from build123d import *

# Parameters (mm, degrees)
SKETCH1_R           = 37.5
SKETCH1_R_2         = 1.5
BOSS_EXTRUDE1_DEPTH = 10
FILLET1_R           = 5


with BuildPart() as part:
    # Sketch1 → Boss-Extrude1 (new body)
    with BuildSketch(Plane(origin=(0, 0, 0), x_dir=(1, 0, 0), z_dir=(0, 1, 0))):
        with Locations(Location((0, 0, 0), (0, 0, 270))):
            Circle(SKETCH1_R)
        with Locations(Location((-24.748737342, -24.748737342, 0), (0, 0, 270))):
            Circle(SKETCH1_R_2, mode=Mode.SUBTRACT)
        with Locations(Location((-9.058666579, -33.80740392, 0), (0, 0, 270))):
            Circle(SKETCH1_R_2, mode=Mode.SUBTRACT)
        with Locations(Location((-33.80740392, -9.058666579, 0), (0, 0, 270))):
            Circle(SKETCH1_R_2, mode=Mode.SUBTRACT)
        with Locations(Location((9.058666579, -33.80740392, 0), (0, 0, 270))):
            Circle(SKETCH1_R_2, mode=Mode.SUBTRACT)
        with Locations(Location((24.748737342, -24.748737342, 0), (0, 0, 270))):
            Circle(SKETCH1_R_2, mode=Mode.SUBTRACT)
        with Locations(Location((33.80740392, -9.058666579, 0), (0, 0, 270))):
            Circle(SKETCH1_R_2, mode=Mode.SUBTRACT)
        with Locations(Location((-33.80740392, 9.058666579, 0), (0, 0, 270))):
            Circle(SKETCH1_R_2, mode=Mode.SUBTRACT)
        with Locations(Location((-24.748737342, 24.748737342, 0), (0, 0, 270))):
            Circle(SKETCH1_R_2, mode=Mode.SUBTRACT)
        with Locations(Location((-9.058666579, 33.80740392, 0), (0, 0, 270))):
            Circle(SKETCH1_R_2, mode=Mode.SUBTRACT)
        with BuildLine():
            ThreePointArc((28.282562779, 10.004830964), (29.567523428, 5.075584529), (30, 0))
            ThreePointArc((30, 0), (29.567523428, -5.075584529), (28.282562779, -10.004830964))
            ThreePointArc((28.282562779, -10.004830964), (30.612711145, -12.034355354), (31.480762114, -15))
            ThreePointArc((31.480762114, -15), (28.509325321, -19.884298118), (22.805719165, -19.491002369))
            ThreePointArc((22.805719165, -19.491002369), (15, -25.980762114), (5.476843614, -29.495833333))
            ThreePointArc((5.476843614, -29.495833333), (5.494207854, -29.747650913), (5.5, -30))
            ThreePointArc((5.5, -30), (-0.252349087, -35.494207854), (-5.476843614, -29.495833333))
            ThreePointArc((-5.476843614, -29.495833333), (-15, -25.980762114), (-22.805719165, -19.491002369))
            ThreePointArc((-22.805719165, -19.491002369), (-30.743901834, -17.75), (-28.282562779, -10.004830964))
            ThreePointArc((-28.282562779, -10.004830964), (-30, 0), (-28.282562779, 10.004830964))
            ThreePointArc((-28.282562779, 10.004830964), (-30.743901834, 17.75), (-22.805719165, 19.491002369))
            ThreePointArc((-22.805719165, 19.491002369), (-15, 25.980762114), (-5.476843614, 29.495833333))
            ThreePointArc((-5.476843614, 29.495833333), (-0.252349087, 35.494207854), (5.5, 30))
            ThreePointArc((5.5, 30), (5.494207854, 29.747650913), (5.476843614, 29.495833333))
            ThreePointArc((5.476843614, 29.495833333), (15, 25.980762114), (22.805719165, 19.491002369))
            ThreePointArc((22.805719165, 19.491002369), (28.509325321, 19.884298118), (31.480762114, 15))
            ThreePointArc((31.480762114, 15), (30.612711145, 12.034355354), (28.282562779, 10.004830964))
        make_face(mode=Mode.SUBTRACT)
        with Locations(Location((33.80740392, 9.058666579, 0), (0, 0, 270))):
            Circle(SKETCH1_R_2, mode=Mode.SUBTRACT)
        with Locations(Location((9.058666579, 33.80740392, 0), (0, 0, 270))):
            Circle(SKETCH1_R_2, mode=Mode.SUBTRACT)
        with Locations(Location((24.748737342, 24.748737342, 0), (0, 0, 270))):
            Circle(SKETCH1_R_2, mode=Mode.SUBTRACT)
    extrude(amount=BOSS_EXTRUDE1_DEPTH)

    # Fillet1
    fillet1_edges = [part.edges().sort_by_distance(p)[0] for p in [
        (-28.282562779, 5, -10.004830964),
        (-28.282562779, 5, 10.004830964),
        (-22.805719165, 5, 19.491002369),
        (-5.476843614, 5, 29.495833333),
        (5.476843614, 5, 29.495833333),
        (22.805719165, 5, 19.491002369),
        (28.282562779, 5, 10.004830964),
        (28.282562779, 5, -10.004830964),
        (22.805719165, 5, -19.491002369),
        (5.476843614, 5, -29.495833333),
        (-5.476843614, 5, -29.495833333),
        (-22.805719165, 5, -19.491002369),
    ]]
    fillet(fillet1_edges, radius=FILLET1_R)


solid = part.part
Geometry: final body of the model. Coordinates: model frame, mm. Give positions to 0.01 mm unless a question says otherwise; leave off trailing zeros. Loops run counter-clockwise (first coordinate to the right, second up) from the corner with the lowest first, then second, coordinate; pieces in that order, holes last. Notation, with made-up numbers: (63.5, 0) -> (118.5, 0) arc R21 cw to (118.5, 33) -> close; hole circle Ø2 at (26.5, 21). An arc over 180 degrees is marked (long way). Put each result on its own line as item: value.
1. Pull-direction query (Z, two-part tool) for faces 1 (the cylindrical face through (26.01, 4.93, -23.94)), 2 (the flat face through (11.3, 0, -28)); classes: released by +Z, released by -Z, zero draft, split by the parting line, or undercut.
Taken from the geometry:
face 1: undercut
face 2: zero draft
2. Ray query, line 1 along Z through (x, y) = (33, 6.75); line 2 along X through (y, z) = (7, 33.5); line 3 along X through (y, z) = (4.75, 0.5). Return the intervals inside material, ascending. Write a range as [from, to].
Taken from the geometry:
line 1: z = [-17.81, -10.32], [-7.79, 7.79], [10.32, 17.81]
line 2: x = [-16.85, -10.53], [-7.59, -4.24], [4.24, 7.59], [10.53, 16.85]
line 3: x = [-37.5, -30], [30, 37.5]
3. Pin query (flat end, axial travel): P1, Ø2.5, axis at x = 24.75, z = -24.75, coming from the +Y side; P2, Ø6, axis at x = -17, y = 4.5, coming from the +Z side; P3, Ø1.5, axis at y = 8.5, z = 1, coming from the -X side; P4, Ø1.5, axis at y = 3.5, z = -18, coming from the +X side. Return the tip coordinate at first contact, or that it passes through.
Taken from the geometry:
P1: passes through
P2: stops at z = 34.79
P3: stops at x = -37.5
P4: stops at x = 33.3
4. Cut plane B-B (z = 27.5). Return the cut outline in (x, y), plus the area to 3 significant figures.
Taken from the geometry:
outline: (-25.5, 0) -> (-11.99, 0) -> (-11.99, 10) -> (-25.5, 10) -> close; (11.99, 0) -> (25.5, 0) -> (25.5, 10) -> (11.99, 10) -> close
area: 270 mm2
5. Cut plane C-C (y = 1.75). Count the separate pieces of the cut face and the enclosed holes in it, plus the area to 3 significant figures.
Taken from the geometry:
separate pieces: 1
enclosed holes: 13
area: 1,190 mm2
6. Cut plane A-A (x = 0). Return the cut outline in (y, z), plus the area to 3 significant figures.
Taken from the geometry:
outline: (0, -37.5) -> (10, -37.5) -> (10, -35.5) -> (0, -35.5) -> close; (0, 35.5) -> (10, 35.5) -> (10, 37.5) -> (0, 37.5) -> close
area: 40.0 mm2
